For this review, take the finished solid that the model builds, in its own axes (mm). Face numbers are marked on the shaded views. A direction names the side the tool comes from. Coordinates: 2 decimals unless noted, no trailing zeros. Order: outer loops, then holes, each group sorted by start corner. A loop starts at its lowest first (then second) coordinate and runs counter-clockwise, first axis right, second up. Notation, with made-up numbers: (-24, 45.25) -> (0, 45.25) arc R21 ccw to (0, 78.25) -> close; hole circle Ø4 at (-16.5, -36.5). An arc over 180 degrees is marked (long way). Answer as a JSON object with one key per item and string values. Group by question number.
1) Wall thickness on L1, parallel to Z at x = -38, y = 1.5; L2, parallel to X at y = 3.45, z = -53; L3, parallel to X at y = 4.75, z = -52: over which ranges is each line inside the solid? List them lowest first.
2) For pin 1 (2.5 mm diameter, centred on x = -38, z = -13, fed in from +Y); pin 2 (0.5 mm diameter, centred on y = 5.5, z = -46.5, fed in from -X); pin 3 (9.5 mm diameter, centred on x = -3.5, z = -27, fed in from +Y), all flat-tipped, find the tip position at first contact; note any pin that passes through.
3) Add section B-B, the plane x = -4. Write out the cut boundary in (y, z), then the cut area to 3 significant figures.
4) Add section A-A, the plane z = -53. Write out the cut boundary in (x, y).
5) Machinability: for the marked faces 1, 2 and 3, which of the approach directions +Z, -Z, +X, -X, +Y, -Y give a long, thin tool a straight path to every point of the face, cutting with its end or side? Answer none if there is none.
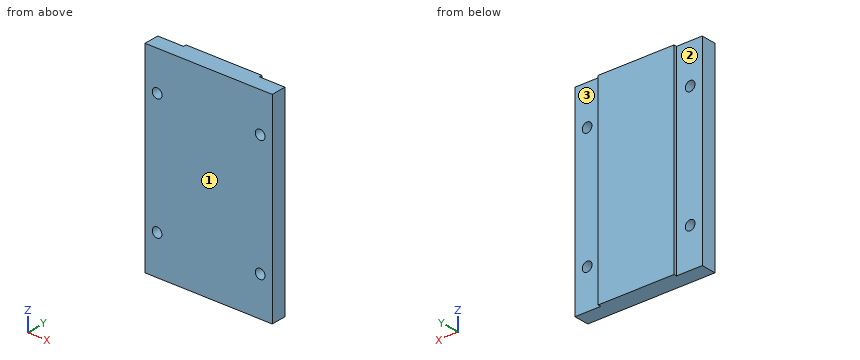
Autodesk Inventor part; units mm, degrees
ref_plane "YZ Plane" through (0, 0, 0) normal (1, 0, 0) x (0, 1, 0)
ref_plane "XZ Plane" through (0, 0, 0) normal (0, 1, 0) x (-1, 0, 0)
ref_plane "XY Plane" through (0, 0, 0) normal (0, 0, 1) x (1, 0, 0)
sketch "スケッチ1" plane through (0, 0, 0) normal (0, 1, 0) x (-1, 0, 0)
  line L0 (0, 0) -> (42, 0)
  line L1 (42, 0) -> (42, -66)
  line L2 (42, -66) -> (0, -66)
  line L3 (0, -66) -> (0, 0)
  dimension "d0" = 42
  dimension "d1" = 66
extrude "押し出し1" add sketch "スケッチ1" along normal blind 5
sketch "スケッチ2" plane through (0, 5, 0) normal (0, 1, 0) x (1, 0, 0)
  line L0 (0, 66) -> (-42, 66)
  line L1 (-33.5, 0) -> (-8.5, 0)
  line L2 (-8.5, 0) -> (-8.5, 66)
  line L3 (-8.5, 66) -> (-33.5, 66)
  line L4 (-33.5, 66) -> (-33.5, 0)
  line L5 (-42, 66) -> (-42, 0)
  point P0 (0, 0)
  dimension "d4" = 25
  dimension "d5" = 8.5
extrude "押し出し2" add sketch "スケッチ2" along normal blind 1
sketch "スケッチ3" plane through (0, 0, 0) normal (0, -1, 0) x (1, 0, 0)
  line L0 (0, 0) -> (0, -66)
  line L1 (0, -66) -> (-42, -66)
  point P0 (-4, -13)
  point P1 (-4, -53)
  point P2 (-38, -53)
  point P3 (-38, -13)
  dimension "d8" = 40
  dimension "d10" = 4
  dimension "d11" = 13
hole "穴1" at (-4, 0, -13) at (-4, 0, -53) at (-38, 0, -53) at (-38, 0, -13) direction (0, 1, 0) diameter 3.2 depth 30 tip angle 118
properties part number "slider_move_gaba" material "アルミニウム 6061-AHC"
Output values:
{
 "1": {"L1": "z = -66 to -54.6, -51.4 to -14.6, -11.4 to 0", "L2": "x = -42 to -39.6, -36.4 to -5.6, -2.4 to 0", "L3": "x = -42 to -39.25, -36.75 to -5.25, -2.75 to 0"},
 "2": {"pin 1": "passes through", "pin 2": "stops at x = -33.5", "pin 3": "stops at y = 5"},
 "3": {"outline": "(0, -66) -> (5, -66) -> (5, -54.6) -> (0, -54.6) -> close; (0, -51.4) -> (5, -51.4) -> (5, -14.6) -> (0, -14.6) -> close; (0, -11.4) -> (5, -11.4) -> (5, 0) -> (0, 0) -> close", "area": "298 mm²"},
 "4": {"outline": "(-42, 0) -> (-39.6, 0) -> (-39.6, 5) -> (-42, 5) -> close; (-36.4, 0) -> (-5.6, 0) -> (-5.6, 5) -> (-8.5, 5) -> (-8.5, 6) -> (-33.5, 6) -> (-33.5, 5) -> (-36.4, 5) -> close; (-2.4, 0) -> (0, 0) -> (0, 5) -> (-2.4, 5) -> close"},
 "5": {"face 1": "+Z, -Z, +X, -X, -Y", "face 2": "+Z, -Z, -X, +Y", "face 3": "+Z, -Z, +X, +Y"}
}
